Geometry check sheet. Reference: the model listing, model coordinates, mm. A direction names the side the tool comes from. Give positions to 0.01 mm unless a question says otherwise; leave off trailing zeros. Order: outer loops, then holes, each group sorted by start corner. A loop starts at its lowest first (then second) coordinate and runs counter-clockwise, first axis right, second up. Notation, with made-up numbers: M 34.5,86 L 67.5,86 A36 cw 67.5,124 Z; hole C -16.5,-12.75 d2. An arc over 180 degrees is marked long. Answer as CSV lines item,"result".
from build123d import *

# Parameters (mm, degrees)
F0_R     = 3.4
F1_DEPTH = 25


with BuildPart() as f1:
    # F0 (on Right) → F1 (new body)
    with BuildSketch(Plane.YZ):
        with BuildLine():
            Line((4.085178, -16.514598), (4.085178, -18.514598))
            ThreePointArc((4.085178, -18.514598), (4.524518, -19.575258), (5.585178, -20.014598))
            Line((5.585178, -20.014598), (16.085178, -20.014598))
            ThreePointArc((16.085178, -20.014598), (18.913605, -18.843025), (20.085178, -16.014598))
            Line((20.085178, -16.014598), (20.085178, -5.514598))
            ThreePointArc((20.085178, -5.514598), (19.645838, -4.453938), (18.585178, -4.014598))
            Line((18.585178, -4.014598), (16.585178, -4.014598))
            ThreePointArc((16.585178, -4.014598), (15.878071, -4.307491), (15.585178, -5.014598))
            Line((15.585178, -5.014598), (15.585178, -6.764598))
            ThreePointArc((15.585178, -6.764598), (15.658401, -6.941375), (15.835178, -7.014598))
            Line((15.835178, -7.014598), (17.835178, -7.014598))
            ThreePointArc((17.835178, -7.014598), (18.011955, -7.087821), (18.085178, -7.264598))
            Line((18.085178, -7.264598), (18.085178, -7.514598))
            ThreePointArc((18.085178, -7.514598), (17.352945, -9.282365), (15.585178, -10.014598))
            Line((15.585178, -10.014598), (14.805538, -10.014598))
            ThreePointArc((14.805538, -10.014598), (14.168971, -9.910589), (13.598613, -9.609381))
            ThreePointArc((13.598613, -9.609381), (10.934174, -7.278628), (8.625654, -4.594903))
            ThreePointArc((8.625654, -4.594903), (8.037936, -3.465013), (7.835178, -2.207654))
            Line((7.835178, -2.207654), (7.835178, 2.178458))
            ThreePointArc((7.835178, 2.178458), (8.037936, 3.435818), (8.625654, 4.565707))
            ThreePointArc((8.625654, 4.565707), (10.934174, 7.249432), (13.598613, 9.580185))
            ThreePointArc((13.598613, 9.580185), (14.168971, 9.881393), (14.805538, 9.985402))
            Line((14.805538, 9.985402), (15.585178, 9.985402))
            ThreePointArc((15.585178, 9.985402), (17.352945, 9.253169), (18.085178, 7.485402))
            Line((18.085178, 7.485402), (18.085178, 7.235402))
            ThreePointArc((18.085178, 7.235402), (18.011955, 7.058625), (17.835178, 6.985402))
            Line((17.835178, 6.985402), (15.835178, 6.985402))
            ThreePointArc((15.835178, 6.985402), (15.658401, 6.912179), (15.585178, 6.735402))
            Line((15.585178, 6.735402), (15.585178, 4.985402))
            ThreePointArc((15.585178, 4.985402), (15.878071, 4.278295), (16.585178, 3.985402))
            Line((16.585178, 3.985402), (18.585178, 3.985402))
            ThreePointArc((18.585178, 3.985402), (19.645838, 4.424742), (20.085178, 5.485402))
            Line((20.085178, 5.485402), (20.085178, 15.985402))
            ThreePointArc((20.085178, 15.985402), (18.913605, 18.813829), (16.085178, 19.985402))
            Line((16.085178, 19.985402), (5.585178, 19.985402))
            ThreePointArc((5.585178, 19.985402), (4.524518, 19.546062), (4.085178, 18.485402))
            Line((4.085178, 18.485402), (4.085178, 16.485402))
            ThreePointArc((4.085178, 16.485402), (4.378071, 15.778295), (5.085178, 15.485402))
            Line((5.085178, 15.485402), (6.835178, 15.485402))
            ThreePointArc((6.835178, 15.485402), (7.011955, 15.558625), (7.085178, 15.735402))
            Line((7.085178, 15.735402), (7.085178, 17.735402))
            ThreePointArc((7.085178, 17.735402), (7.158401, 17.912179), (7.335178, 17.985402))
            Line((7.335178, 17.985402), (7.585178, 17.985402))
            ThreePointArc((7.585178, 17.985402), (9.352945, 17.253169), (10.085178, 15.485402))
            Line((10.085178, 15.485402), (10.085178, 14.705762))
            ThreePointArc((10.085178, 14.705762), (9.981169, 14.069195), (9.67996, 13.498837))
            ThreePointArc((9.67996, 13.498837), (7.349208, 10.834398), (4.665483, 8.525878))
            ThreePointArc((4.665483, 8.525878), (3.535593, 7.93816), (2.278234, 7.735402))
            Line((2.278234, 7.735402), (-2.107878, 7.735402))
            ThreePointArc((-2.107878, 7.735402), (-3.365238, 7.93816), (-4.495127, 8.525878))
            ThreePointArc((-4.495127, 8.525878), (-7.178852, 10.834398), (-9.509605, 13.498837))
            ThreePointArc((-9.509605, 13.498837), (-9.810813, 14.069195), (-9.914822, 14.705762))
            Line((-9.914822, 14.705762), (-9.914822, 15.485402))
            ThreePointArc((-9.914822, 15.485402), (-9.182589, 17.253169), (-7.414822, 17.985402))
            Line((-7.414822, 17.985402), (-7.164822, 17.985402))
            ThreePointArc((-7.164822, 17.985402), (-6.988045, 17.912179), (-6.914822, 17.735402))
            Line((-6.914822, 17.735402), (-6.914822, 15.735402))
            ThreePointArc((-6.914822, 15.735402), (-6.841599, 15.558625), (-6.664822, 15.485402))
            Line((-6.664822, 15.485402), (-4.914822, 15.485402))
            ThreePointArc((-4.914822, 15.485402), (-4.207715, 15.778295), (-3.914822, 16.485402))
            Line((-3.914822, 16.485402), (-3.914822, 18.485402))
            ThreePointArc((-3.914822, 18.485402), (-4.354162, 19.546062), (-5.414822, 19.985402))
            Line((-5.414822, 19.985402), (-15.914822, 19.985402))
            ThreePointArc((-15.914822, 19.985402), (-18.743249, 18.813829), (-19.914822, 15.985402))
            Line((-19.914822, 15.985402), (-19.914822, 5.485402))
            ThreePointArc((-19.914822, 5.485402), (-19.475482, 4.424742), (-18.414822, 3.985402))
            Line((-18.414822, 3.985402), (-16.414822, 3.985402))
            ThreePointArc((-16.414822, 3.985402), (-15.707715, 4.278295), (-15.414822, 4.985402))
            Line((-15.414822, 4.985402), (-15.414822, 6.735402))
            ThreePointArc((-15.414822, 6.735402), (-15.488045, 6.912179), (-15.664822, 6.985402))
            Line((-15.664822, 6.985402), (-17.664822, 6.985402))
            ThreePointArc((-17.664822, 6.985402), (-17.841599, 7.058625), (-17.914822, 7.235402))
            Line((-17.914822, 7.235402), (-17.914822, 7.485402))
            ThreePointArc((-17.914822, 7.485402), (-17.182589, 9.253169), (-15.414822, 9.985402))
            Line((-15.414822, 9.985402), (-14.635182, 9.985402))
            ThreePointArc((-14.635182, 9.985402), (-13.998616, 9.881393), (-13.428257, 9.580185))
            ThreePointArc((-13.428257, 9.580185), (-10.763818, 7.249432), (-8.455298, 4.565707))
            ThreePointArc((-8.455298, 4.565707), (-7.86758, 3.435818), (-7.664822, 2.178458))
            Line((-7.664822, 2.178458), (-7.664822, -2.207654))
            ThreePointArc((-7.664822, -2.207654), (-7.86758, -3.465013), (-8.455298, -4.594903))
            ThreePointArc((-8.455298, -4.594903), (-10.763818, -7.278628), (-13.428257, -9.609381))
            ThreePointArc((-13.428257, -9.609381), (-13.998616, -9.910589), (-14.635182, -10.014598))
            Line((-14.635182, -10.014598), (-15.414822, -10.014598))
            ThreePointArc((-15.414822, -10.014598), (-17.182589, -9.282365), (-17.914822, -7.514598))
            Line((-17.914822, -7.514598), (-17.914822, -7.264598))
            ThreePointArc((-17.914822, -7.264598), (-17.841599, -7.087821), (-17.664822, -7.014598))
            Line((-17.664822, -7.014598), (-15.664822, -7.014598))
            ThreePointArc((-15.664822, -7.014598), (-15.488045, -6.941375), (-15.414822, -6.764598))
            Line((-15.414822, -6.764598), (-15.414822, -5.014598))
            ThreePointArc((-15.414822, -5.014598), (-15.707715, -4.307491), (-16.414822, -4.014598))
            Line((-16.414822, -4.014598), (-18.414822, -4.014598))
            ThreePointArc((-18.414822, -4.014598), (-19.475482, -4.453938), (-19.914822, -5.514598))
            Line((-19.914822, -5.514598), (-19.914822, -16.014598))
            ThreePointArc((-19.914822, -16.014598), (-18.743249, -18.843025), (-15.914822, -20.014598))
            Line((-15.914822, -20.014598), (-5.414822, -20.014598))
            ThreePointArc((-5.414822, -20.014598), (-4.354162, -19.575258), (-3.914822, -18.514598))
            Line((-3.914822, -18.514598), (-3.914822, -16.514598))
            ThreePointArc((-3.914822, -16.514598), (-4.207715, -15.807491), (-4.914822, -15.514598))
            Line((-4.914822, -15.514598), (-6.664822, -15.514598))
            ThreePointArc((-6.664822, -15.514598), (-6.841599, -15.587821), (-6.914822, -15.764598))
            Line((-6.914822, -15.764598), (-6.914822, -17.764598))
            ThreePointArc((-6.914822, -17.764598), (-6.988045, -17.941375), (-7.164822, -18.014598))
            Line((-7.164822, -18.014598), (-7.414822, -18.014598))
            ThreePointArc((-7.414822, -18.014598), (-9.182589, -17.282365), (-9.914822, -15.514598))
            Line((-9.914822, -15.514598), (-9.914822, -14.734958))
            ThreePointArc((-9.914822, -14.734958), (-9.810813, -14.098391), (-9.509605, -13.528033))
            ThreePointArc((-9.509605, -13.528033), (-7.178852, -10.863594), (-4.495127, -8.555074))
            ThreePointArc((-4.495127, -8.555074), (-3.365238, -7.967356), (-2.107878, -7.764598))
            Line((-2.107878, -7.764598), (2.278234, -7.764598))
            ThreePointArc((2.278234, -7.764598), (3.535593, -7.967356), (4.665483, -8.555074))
            ThreePointArc((4.665483, -8.555074), (7.349208, -10.863594), (9.67996, -13.528033))
            ThreePointArc((9.67996, -13.528033), (9.981169, -14.098391), (10.085178, -14.734958))
            Line((10.085178, -14.734958), (10.085178, -15.514598))
            ThreePointArc((10.085178, -15.514598), (9.352945, -17.282365), (7.585178, -18.014598))
            Line((7.585178, -18.014598), (7.335178, -18.014598))
            ThreePointArc((7.335178, -18.014598), (7.158401, -17.941375), (7.085178, -17.764598))
            Line((7.085178, -17.764598), (7.085178, -15.764598))
            ThreePointArc((7.085178, -15.764598), (7.011955, -15.587821), (6.835178, -15.514598))
            Line((6.835178, -15.514598), (5.085178, -15.514598))
            ThreePointArc((5.085178, -15.514598), (4.378071, -15.807491), (4.085178, -16.514598))
        make_face()
        with Locations((0.085178, -0.014598)):
            Circle(F0_R, mode=Mode.SUBTRACT)
    extrude(amount=-F1_DEPTH)


solid = f1.part
(1) Tool access check on faces 4 (the face through (0, 0, 5)), 5 (the face through (-12, 18, 3.985)), 6 (the face through (-12, 17, -7.015)), 7 (the face through (-12.325, -18.712, 18.845)), 8 (the face through (-12, 0, -7.765)). Record the directions out of +Z, -Z, +X, -X, +Y, -Y that give a thin tool (end or side, any length) a straight path to the whole face; none if there is none.
The answers:
face 4,"+Z, -Z, +X, +Y, -Y"
face 5,"+X, -X, +Y"
face 6,"+X, -X"
face 7,"+Z, +X, -X, -Y"
face 8,"-Z, +X, -X"
(2) Section check B-B on z = 17. Enter the section's corners in (x, y), then the cut area to 3 significant figures.
The answers:
outline,"M -25,-19.78 L 0,-19.78 L 0,-9.4 L -25,-9.4 Z; M -25,-6.91 L 0,-6.91 L 0,-3.91 L -25,-3.91 Z; M -25,4.09 L 0,4.09 L 0,7.09 L -25,7.09 Z; M -25,9.57 L 0,9.57 L 0,19.95 L -25,19.95 Z"
area,"669 mm2"
(3) Draft check along Z on faces 1 (the face through (-12.32, -4.37, -19.59)), 2 (the face through (-12.325, 10.969, -7.314)), 3 (the face through (-12, 4.085, -18)). Enter one of: +Z half, -Z half, draft (parallel to the pull), parting line (faces both ways), or undercut.
The answers:
face 1,"-Z half"
face 2,"undercut"
face 3,"draft"
(4) Gauge pin test, flat ends, axial feed: P1, Ø0.6, axis at x = -9.5, y = -16.5, coming from the -Z side; P2, Ø0.6, axis at x = -11.5, y = -16.5, coming from the +Z side; P3, Ø3, axis at x = -3.5, y = 0.5, coming from the -Z side. Record the tip position at first contact, or that the pin passes through.
The answers:
P1,"stops at z = -20"
P2,"stops at z = 19.98"
P3,"stops at z = -7.76"
(5) Section check C-C on y = -10.5. Enter the section's corners in (x, z).
The answers:
outline,"M -25,-20.01 L 0,-20.01 L 0,-7.01 L -25,-7.01 Z; M -25,6.98 L 0,6.98 L 0,19.99 L -25,19.99 Z"
(6) Section check A-A on z = 1. Enter the section's corners in (x, y), then the cut area to 3 significant figures.
The answers:
outline,"M -25,-7.66 L 0,-7.66 L 0,-3.16 L -25,-3.16 Z; M -25,3.33 L 0,3.33 L 0,7.84 L -25,7.84 Z"
area,"225 mm2"
(7) Material ranges on line 1 (Y direction, x = -21, z = -5.5); line 2 (Y direction, x = -1.75, z = 15); line 3 (Z direction, x = -0.75, y = -5), recorded low to high.
The answers:
line 1,"y = -19.91 to -15.41, -9.16 to 9.33, 15.59 to 20.09"
line 2,"y = -19.91 to -9.91, 10.09 to 20.09"
line 3,"z = -19.96 to -15.51, -8.94 to 8.91, 15.49 to 19.93"
